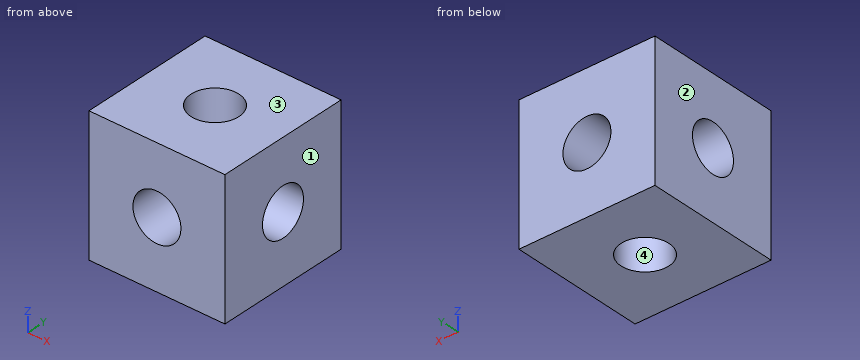
Autodesk Fusion 360 part; units mm, degrees
sketch "草图1" plane through (0, 0, 0) normal (0, 0, 1) x (1, 0, 0)
  line L0 (0, 0) -> (10, 0)
  line L1 (10, 0) -> (10, 10)
  line L2 (10, 10) -> (0, 10)
  line L3 (0, 10) -> (0, 0)
extrude "拉伸1" add sketch "草图1" along normal blind 10
hole "孔1" at (5, 5, 10) direction (0, 0, -1) diameter 3.529 depth 10 tip angle 180
hole "孔2" at (0, 5, 5) direction (1, 0, 0) diameter 3.529 depth 5 tip angle 180
hole "孔3" at (10, 5, 5) direction (-1, 0, 0) diameter 3.529 depth 5 tip angle 180
hole "孔4" at (5, 10, 5) direction (0, -1, 0) diameter 3.529 depth 5 tip angle 180
hole "孔5" at (5, 0, 5) direction (0, 1, 0) diameter 3.529 depth 5 tip angle 180
The listing builds one solid part. Answer for the finished solid, in the listing's coordinates (mm). Face numbers are marked on the shaded views. Coordinates: 2 decimals unless noted, no trailing zeros. Write each loop counter-clockwise with the first axis right and the second up, starting at its lowest first coordinate (ties: lowest second). Pieces come first, ordered by that corner, then holes. Notation, with made-up numbers: (-29, 45.5) - (-7, 45.5) arc R27 ccw to (-7, 84.5) - close; hole circle Ø11 at (73, 32.25). An arc over 180 degrees is marked (long way). Return JSON: item names as keys, results as strings.
1. Consider line 1 along Z through (x, y) = (2, 5); line 2 along X through (y, z) = (3.75, 6.5). Determine where each line is inside the solid, lowest interval first.
Final values:
{"line 1": "0 to 3.24, 6.76 to 10", "line 2": "0 to 3.75, 6.25 to 10"}
2. The part is cut by section C-C on y = 2.25. Determine the outline of the cut face in (x, z).
Final values:
{"outline": "(0, 0) - (10, 0) - (10, 10) - (0, 10) - close; hole circle Ø3.53 at (5, 5)"}
3. For a pull along X with two mould halves and no side action, classify the marked faces 1, 2, 3 and 4 as +X half, -X half, draft (parallel to the pull), parting line (faces both ways), or undercut.
Final values:
{"face 1": "+X half", "face 2": "-X half", "face 3": "draft", "face 4": "undercut"}
4. The part is cut by section A-A on x = 5. Determine the outline of the cut face in (y, z), then the cut area to 3 significant figures.
Final values:
{"outline": "(0, 0) - (3.24, 0) - (3.24, 3.24) - (0, 3.24) - close; (0, 6.76) - (3.24, 6.76) - (3.24, 10) - (0, 10) - close; (6.76, 0) - (10, 0) - (10, 3.24) - (6.76, 3.24) - close; (6.76, 6.76) - (10, 6.76) - (10, 10) - (6.76, 10) - close", "area": "41.9 mm^2"}
